from build123d import *

# Parameters (mm, degrees)
SKETCH1_R           = 1
BOSS_EXTRUDE1_DEPTH = 10
SKETCH2_R           = 2.5
BOSS_EXTRUDE2_DEPTH = 1.5
FILLET1_R           = 1
CUT_EXTRUDE1_DEPTH  = 1


with BuildPart() as part:
    # Sketch1 → Boss-Extrude1 (new body)
    with BuildSketch(Plane(origin=(0, 0, 0), x_dir=(1, 0, 0), z_dir=(0, 1, 0))):
        with Locations(Location((0, 0, 0), (0, 0, 270))):
            Circle(SKETCH1_R)
    extrude(amount=BOSS_EXTRUDE1_DEPTH)

    # Sketch2 → Boss-Extrude2 (add)
    with BuildSketch(Plane(origin=(0, 10, 0), x_dir=(1, 0, 0), z_dir=(0, 1, 0))):
        with Locations(Location((0, 0, 0), (0, 0, 270))):
            Circle(SKETCH2_R)
    extrude(amount=BOSS_EXTRUDE2_DEPTH)

    # Fillet1
    fillet1_edges = [part.edges().sort_by_distance(p)[0] for p in [
        (0, 11.5, -2.5),
    ]]
    fillet(fillet1_edges, radius=FILLET1_R)

    # Sketch3 → Cut-Extrude1 (cut)
    with BuildSketch(Plane(origin=(0, 11.5, 0), x_dir=(1, 0, 0), z_dir=(0, 1, 0))):
        with BuildLine():
            Line((-0.4, 0.6), (-0.4, 1.369908904))
            ThreePointArc((-0.4, 1.369908904), (-0.341421356, 1.51133026), (-0.2, 1.569908904))
            Line((-0.2, 1.569908904), (0.2, 1.569908904))
            ThreePointArc((0.2, 1.569908904), (0.341421356, 1.51133026), (0.4, 1.369908904))
            Line((0.4, 1.369908904), (0.4, 0.6))
            ThreePointArc((0.4, 0.6), (0.458578644, 0.458578644), (0.6, 0.4))
            Line((0.6, 0.4), (1.37, 0.4))
            ThreePointArc((1.37, 0.4), (1.511421356, 0.341421356), (1.57, 0.2))
            Line((1.57, 0.2), (1.57, -0.2))
            ThreePointArc((1.57, -0.2), (1.511421356, -0.341421356), (1.37, -0.4))
            Line((1.37, -0.4), (0.6, -0.4))
            ThreePointArc((0.6, -0.4), (0.458578644, -0.458578644), (0.4, -0.6))
            Line((0.4, -0.6), (0.4, -1.369908904))
            ThreePointArc((0.4, -1.369908904), (0.341421356, -1.51133026), (0.2, -1.569908904))
            Line((0.2, -1.569908904), (-0.2, -1.569908904))
            ThreePointArc((-0.2, -1.569908904), (-0.341421356, -1.51133026), (-0.4, -1.369908904))
            Line((-0.4, -1.369908904), (-0.4, -0.6))
            ThreePointArc((-0.4, -0.6), (-0.458578644, -0.458578644), (-0.6, -0.4))
            Line((-0.6, -0.4), (-1.37, -0.4))
            ThreePointArc((-1.37, -0.4), (-1.511421356, -0.341421356), (-1.57, -0.2))
            Line((-1.57, -0.2), (-1.57, 0.2))
            ThreePointArc((-1.57, 0.2), (-1.511421356, 0.341421356), (-1.37, 0.4))
            Line((-1.37, 0.4), (-0.6, 0.4))
            ThreePointArc((-0.6, 0.4), (-0.458578644, 0.458578644), (-0.4, 0.6))
        make_face()
    extrude(amount=-CUT_EXTRUDE1_DEPTH, mode=Mode.SUBTRACT)


solid = part.part
Geometry check sheet. Reference: the model listing, model coordinates, mm. A direction names the side the tool comes from. Round coordinates to 2 decimals unless told otherwise and drop trailing zeros. Order: outer loops, then holes, each group sorted by start corner. A loop starts at its lowest first (then second) coordinate and runs counter-clockwise, first axis right, second up. Notation, with made-up numbers: M 86.5,-4.75 L 102.5,-4.75 A18 ccw 102.5,9.25 Z; hole C 51.5,75.5 d4. An arc over 180 degrees is marked long. Answer in a Markdown table with one row per item. Add a question column.
Item 1: Depth check by flat-ended pin: pin 1 Ø1.5 at (x, y) = (-0.5, 3.5) entering from -Z; pin 2 Ø0.6 at (y, z) = (11, 1) entering from +X; pin 3 Ø0.6 at (x, y) = (1, 11) entering from -Z. Enter the tip coordinate at first touch or a pass-through.
Item 2: Set-up check for faces 4 (the face through (-1, 5, 0)), 5 (the face through (0.8, 11.5, -0.8)): record each of +Z, -Z, +X, -X, +Y, -Y from which the full face is reachable in a straight line by a thin tool's end or side.
Item 3: Sectioned sample at B-B, the plane z = 0. Enter the section's corners in (x, y), plus the area to 3 significant figures.
Item 4: Sectioned sample at A-A, the plane x = 0. Enter the section's corners in (y, z).
Item 5: Sectioned sample at C-C, the plane y = 5.5. Enter the section's corners in (x, z).
Item 6: Material ranges on L1, parallel to Y at x = 0.25, z = 0.4; L2, parallel to Y at x = 1.15, z = -0.3; L3, parallel to Z at x = 0.9, y = 8, recorded low to high. Write a range as [from, to].
Item 7: Draft check along Z on faces 1 (the face through (-0.8, 11.5, 0.8)), 2 (the face through (0, 10.5, 0)), 3 (the face through (-2.44, 10.25, -0.54)). Enter one of: released by +Z, released by -Z, zero draft, split by the parting line, or undercut.
Filled in:
| question | item | result |
|---|---|---|
| 1 | pin 1 | stops at z = -1 |
| 1 | pin 2 | stops at x = 2.33 |
| 1 | pin 3 | stops at z = -2.33 |
| 2 | face 4 | -Y |
| 2 | face 5 | +Z, -Z, +X, -X, +Y |
| 3 | outline | M -2.5,10 L -1,10 L -1,0 L 1,0 L 1,10 L 2.5,10 L 2.5,10.5 A1 ccw 1.57,11.5 L 1.57,10.5 L -1.57,10.5 L -1.57,11.5 A1 ccw -2.5,10.5 Z |
| 3 | area | 23.9 mm² |
| 4 | outline | M 0,-1 L 10,-1 L 10,-2.5 L 10.5,-2.5 A1 ccw 11.5,-1.57 L 10.5,-1.57 L 10.5,1.57 L 11.5,1.57 A1 ccw 10.5,2.5 L 10,2.5 L 10,1 L 0,1 Z |
| 5 | outline | C 0,0 d2 |
| 6 | L1 | y = [0, 10.5] |
| 6 | L2 | y = [10, 10.5] |
| 6 | L3 | z = [-0.44, 0.44] |
| 7 | face 1 | zero draft |
| 7 | face 2 | undercut |
| 7 | face 3 | split by the parting line |
